CAD build for the part. Positions are in the model's coordinates, mm. A direction names the side the tool comes from. Give positions to 0.01 mm unless a question says otherwise; leave off trailing zeros. Order: outer loops, then holes, each group sorted by start corner. A loop starts at its lowest first (then second) coordinate and runs counter-clockwise, first axis right, second up. Notation, with made-up numbers: (28, 4.5) -> (58, 4.5) arc R27 cw to (58, 37.5) -> close; hole circle Ø8 at (59.25, 9). An arc over 180 degrees is marked (long way). Answer as CSV lines item,"result".
```python
from build123d import *

# Parameters (mm, degrees)
F1_DEPTH = 762


with BuildPart() as f1:
    # F0 (on Front) → F1 (new body)
    with BuildSketch(Plane.XZ):
        with BuildLine():
            Line((-31.499875, 80.088559), (-31.499875, 72.680225))
            Line((-31.499875, 72.680225), (-31.499875, -72.311441))
            Line((-31.499875, -72.311441), (17.268125, -72.311441))
            Line((17.268125, -72.311441), (17.268125, -69.949241))
            ThreePointArc((17.268125, -69.949241), (15.408253, -65.459113), (10.918125, -63.599241))
            Line((10.918125, -63.599241), (-26.419875, -63.599241))
            Line((-26.419875, -63.599241), (-26.419875, 71.376359))
            Line((-26.419875, 71.376359), (10.918125, 71.376359))
            ThreePointArc((10.918125, 71.376359), (15.408253, 73.236231), (17.268125, 77.726359))
            Line((17.268125, 77.726359), (17.268125, 80.088559))
            Line((17.268125, 80.088559), (-31.499875, 80.088559))
        make_face()
    extrude(amount=F1_DEPTH)


solid = f1.part
```
1) Pin check, flat tip, straight feed: P1, Ø10, axis at y = -204.5, z = 58, coming from the +X side. Stop position of the tip, or through.
Data:
P1,"stops at x = -26.42"
2) Which spindle directions (+Z, -Z, +X, -X, +Y, -Y) get a long thin tool onto all of the face, cutting with end or side? Do faces 1 (the flat face through (-7, -376, -63.599)), 2 (the flat face through (-27, 0, 16)). Say none if no direction does.
Data:
face 1,"+X, +Y, -Y"
face 2,"+Z, -Z, +X, -X, +Y"
3) Band-saw the part on A-A, the plane x = -0.5. Write the cut outline in (y, z).
Data:
outline,"(-762, -72.31) -> (0, -72.31) -> (0, -63.6) -> (-762, -63.6) -> close; (-762, 71.38) -> (0, 71.38) -> (0, 80.09) -> (-762, 80.09) -> close"
4) Wall check: line 1 along Z through (x, y) = (7, -439.5); line 2 along X through (y, z) = (-674, 12.5). Give the ranges that are in metal, low to high. Write a range as [from, to].
Data:
line 1,"z = [-72.31, -63.6], [71.38, 80.09]"
line 2,"x = [-31.5, -26.42]"
5) Band-saw the part on C-C, the plane z = 22. Write the cut outline in (x, y), then the cut area to 3 significant figures.
Data:
outline,"(-31.5, -762) -> (-26.42, -762) -> (-26.42, 0) -> (-31.5, 0) -> close"
area,"3,870 mm2"
6) Pull direction Z, two halves, no side cores. Call faces 3 (the flat face through (-26.42, -376, 3)), 4 (the flat face through (-7, -376, -72.311)), 5 (the flat face through (-27, -762, 16)): pulls with the +Z half, pulls with the -Z half, needs draft (parallel to the pull), parting line crosses it, or undercut.
Data:
face 3,"undercut"
face 4,"pulls with the -Z half"
face 5,"needs draft"
7) Band-saw the part on B-B, the plane y = -461. Write the cut outline in (x, z).
Data:
outline,"(-31.5, -72.31) -> (17.27, -72.31) -> (17.27, -69.95) arc R6.35 ccw to (10.92, -63.6) -> (-26.42, -63.6) -> (-26.42, 71.38) -> (10.92, 71.38) arc R6.35 ccw to (17.27, 77.73) -> (17.27, 80.09) -> (-31.5, 80.09) -> close"
